Geometry: final body of the model. Coordinates: model frame, mm. A direction names the side the tool comes from. Give positions to 0.01 mm unless a question says otherwise; leave off trailing zeros. Order: outer loops, then holes, each group sorted by start corner. A loop starts at its lowest first (then second) coordinate and runs counter-clockwise, first axis right, second up. Notation, with made-up numbers: M 24,39.25 L 39,39.25 A19 ccw 39,51.25 Z; hole C 10,-30.75 d9. An arc over 180 degrees is marked long. Use CSV: the item, a comma, the result in double quotes.
```python
from build123d import *

# Parameters (mm, degrees)
SKETCH1_R           = 53.975
BOSS_EXTRUDE1_DEPTH = 11.1125
SKETCH2_R           = 57.15
BOSS_EXTRUDE2_DEPTH = 1.5875
SKETCH3_R           = 47.625
CUT_EXTRUDE1_DEPTH  = 6.35
SKETCH4_R           = 12.7
BOSS_EXTRUDE3_DEPTH = 6.35
CHAMFER2_SIZE       = 1.5875


with BuildPart() as part:
    # Sketch1 → Boss-Extrude1 (new body)
    with BuildSketch(Plane.XY):
        Circle(SKETCH1_R)
    extrude(amount=BOSS_EXTRUDE1_DEPTH)

    # Sketch2 → Boss-Extrude2 (add)
    with BuildSketch(Plane.XY.offset(11.1125)):
        Circle(SKETCH2_R)
    extrude(amount=BOSS_EXTRUDE2_DEPTH)

    # Sketch3 → Cut-Extrude1 (cut)
    with BuildSketch(Plane.XY.offset(12.7)):
        Circle(SKETCH3_R)
    extrude(amount=-CUT_EXTRUDE1_DEPTH, mode=Mode.SUBTRACT)

    # Sketch4 → Boss-Extrude3 (add)
    with BuildSketch(Plane.XY.offset(6.35)):
        Circle(SKETCH4_R)
        Polygon((7.332348419, 0), (3.666174209, 6.35), (-3.666174209, 6.35), (-7.332348419, 0), (-3.666174209, -6.35), (3.666174209, -6.35), align=None, mode=Mode.SUBTRACT)
    extrude(amount=BOSS_EXTRUDE3_DEPTH)

    # Chamfer2
    chamfer2_edges = [part.edges().sort_by_distance(p)[0] for p in [
        (-12.7, 0, 12.7),
    ]]
    chamfer(chamfer2_edges, length=CHAMFER2_SIZE)


solid = part.part
```
1. Reachability of faces 5 (the face through (5, -5, 12.7)), 6 (the face through (42.1, 34.1, 11.112)), 7 (the face through (0, 6.35, 9)) from +Z, -Z, +X, -X, +Y, -Y: full face, straight path, thin tool, end or side. Return the list, or none.
Answer:
face 5,"+Z, +X, -X, +Y, -Y"
face 6,"-Z"
face 7,"+Z"
2. Pin query (flat end, axial travel): pin 1 Ø6 at (y, z) = (10, 5) entering from -X; pin 2 Ø2 at (x, z) = (-40.5, 1.5) entering from +Y; pin 3 Ø3 at (x, y) = (-10.5, -25) entering from +Z. Return the tip coordinate at first contact, or that it passes through.
Answer:
pin 1,"x = -53.52"
pin 2,"y = 36.78"
pin 3,"z = 6.35"
3. Section C-C, the plane z = 1.75. Return the cut outline in (x, y) (3 decimals), plus the area to 3 significant figures.
Answer:
outline,"C 0,0 d107.95"
area,"9,150 mm2"
4. Pull-direction query (X, two-part tool) for faces 1 (the face through (-1, 1, 0)), 2 (the face through (5.474, -3.219, 9.481)), 3 (the face through (-2.75, -12.4, 8.7)), 4 (the face through (-57.095, 2.513, 11.895)); classes: +X half, -X half, draft (parallel to the pull), parting line (faces both ways), or undercut.
Answer:
face 1,"draft"
face 2,"undercut"
face 3,"undercut"
face 4,"parting line"
5. Line query: line 1 (Y direction, x = 0, z = 10.5) (3 decimals); line 2 (Z direction, x = 38, y = -24); line 3 (X direction, y = 27, z = 6.75). Output: solid intervals per line, ascending.
Answer:
line 1,"-53.975 to -47.625, -12.7 to -6.35, 6.35 to 12.7, 47.625 to 53.975"
line 2,"0 to 6.35"
line 3,"-46.74 to -39.23, 39.23 to 46.74"
6. Section B-B, the plane y = 37.5. Return the cut outline in (x, z).
Answer:
outline,"M -43.13,11.11 L -38.82,11.11 L -38.82,0 L 38.82,0 L 38.82,11.11 L 43.13,11.11 L 43.13,12.7 L 29.36,12.7 L 29.36,6.35 L -29.36,6.35 L -29.36,12.7 L -43.13,12.7 Z"
7. Section D-D, the plane y = 24. Return the cut outline in (x, z).
Answer:
outline,"M -51.87,11.11 L -48.35,11.11 L -48.35,0 L 48.35,0 L 48.35,11.11 L 51.87,11.11 L 51.87,12.7 L 41.14,12.7 L 41.14,6.35 L -41.14,6.35 L -41.14,12.7 L -51.87,12.7 Z"
